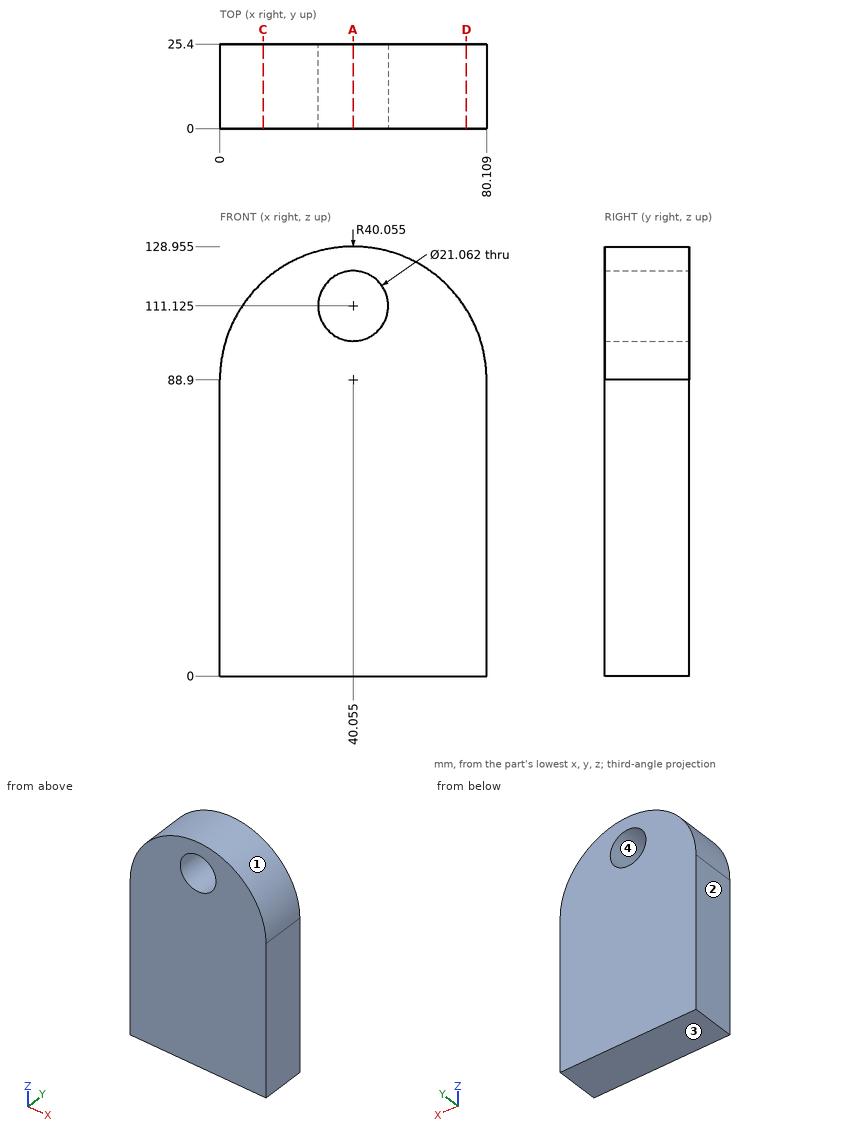
Geometry check sheet. Reference: drawing and pictorial views, mm from the part's lowest x, y, z. Give positions to 0.01 mm unless a question says otherwise; leave off trailing zeros. Write each loop counter-clockwise with the first axis right and the second up, starting at its lowest first coordinate (ties: lowest second). Pieces come first, ordered by that corner, then holes. Notation, with made-up numbers: (-3, 51.25) - (6, 51.25) arc R28 cw to (6, 83.25) - close; hole circle Ø1 at (-11.75, 50). An arc over 180 degrees is marked (long way). Use a Markdown table: item, result.
Q1. Section check A-A, the plane x = 40. Enter the section's corners in (y, z) (1 decimal), then the cut area to 3 significant figures.
Computed:
| item | result |
|---|---|
| outline | (0, 0) - (25.4, 0) - (25.4, 100.6) - (0, 100.6) - close; (0, 121.7) - (25.4, 121.7) - (25.4, 129) - (0, 129) - close |
| area | 2,740 mm² |
Q2. Draft check along Z on the marked faces 1, 2, 3 and 4. Enter one of: pulls with the +Z half, pulls with the -Z half, needs draft (parallel to the pull), parting line crosses it, or undercut.
Computed:
| item | result |
|---|---|
| face 1 | pulls with the +Z half |
| face 2 | needs draft |
| face 3 | pulls with the -Z half |
| face 4 | undercut |
Q3. Go/stop test with flat-tipped pins: P1, Ø2, axis at x = 51, y = 6, coming from the -Z side; P2, Ø4, axis at y = 10.5, z = 109.5, coming from the +X side; P3, Ø12, axis at x = 10, y = 22.5, coming from the +Z side; P4, Ø5, axis at x = 20, y = 4, coming from the +Z side. Record where each tip stops, or that it passes through.
Computed:
| item | result |
|---|---|
| P1 | stops at z = 0 |
| P2 | stops at x = 75.53 |
| P3 | stops at z = 120.93 |
| P4 | stops at z = 124.9 |
Q4. Section check C-C, the plane x = 13. Enter the section's corners in (y, z).
Computed:
| item | result |
|---|---|
| outline | (0, 0) - (25.4, 0) - (25.4, 118.44) - (0, 118.44) - close |
Q5. Section check D-D, the plane x = 74. Enter the section's corners in (y, z), then the cut area to 3 significant figures.
Computed:
| item | result |
|---|---|
| outline | (0, 0) - (25.4, 0) - (25.4, 110.16) - (0, 110.16) - close |
| area | 2,800 mm² |
Q6. Thickness scan on L1, parallel to X at y = 19, z = 114.5; L2, parallel to Z at x = 47, y = 17.5; L3, parallel to Z at x = 71.5, y = 19. Record the ranges inside material, lowest first. Write a range as [from, to].
Computed:
| item | result |
|---|---|
| L1 | x = [9.25, 30.08], [50.03, 70.86] |
| L2 | z = [0, 103.21], [119.04, 128.35] |
| L3 | z = [0, 113.71] |
